Geometry: final body of the model. Coordinates: model frame, mm. A direction names the side the tool comes from. Give positions to 0.01 mm unless a question says otherwise; leave off trailing zeros. Loops run counter-clockwise (first coordinate to the right, second up) from the corner with the lowest first, then second, coordinate; pieces in that order, holes last. Notation, with made-up numbers: (-18, 61.25) -> (-2, 61.25) arc R36 cw to (-2, 99.25) -> close; hole circle Ø2 at (66.25, 63.5). An arc over 180 degrees is marked (long way). One line per question, with ' | ' between items. Start each with the question number.
Item 1: Section B-B on x = 9.5. Return loops of the section in (y, z), then the cut area to 3 significant figures.
Item 2: Section D-D on z = -180. Return loops of the section in (x, y), then the cut area to 3 significant figures.
Item 3: Pin query (flat end, axial travel): P1, Ø1.8, axis at x = -26.5, z = -94, coming from the +Y side; P2, Ø10, axis at y = 37, z = -14.5, coming from the +X side; P3, Ø2, axis at y = 85, z = -59.5, coming from the +X side. Return the tip coordinate at first contact, or that it passes through.
Item 4: Set-up query: faces 1 (the flat face through (7, 56, -137.408)), 2 (the flat face through (-23, 0, 0)). Return all of +Z, -Z, +X, -X, +Y, -Y with unobstructed straight access to the full face (end or side cutting, diameter ignored); none if empty.
Item 5: Section A-A on y = 31. Return loops of the section in (x, z), then the cut area to 3 significant figures.
Item 6: Material intervals for line 1 along X through (y, z) = (23.5, -145.5); line 2 along Y through (x, z) = (-6, -118.5); line 3 along Z through (x, y) = (74, 25.5), sorted ascending. Write a range as [from, to].
Item 7: Section C-C on y = 98. Give the number of separate pieces and of enclosed holes in the cut face, then the cut area to 3 significant figures.
from build123d import *

# Parameters (mm, degrees)
ALUMINUM_BLOCK_DEPTH = 113.03
A_ARM_SKETCHES_R     = 3
A_ARM_HOLES_DEPTH    = 20


with BuildPart() as part:
    # Sketch1 → ALUMINUM BLOCK (new body)
    with BuildSketch(Plane(origin=(0, 0, 0), x_dir=(1, 0, 0), z_dir=(0, 1, 0))):
        Polygon((-187.5, -135.642424533), (244.3, -135.642424533), (244.3, -46.742424533), (98.25, 137.407575467), (-85.9, 137.407575467), (-85.9, 207.257575467), (-187.5, 207.257575467), align=None)
    extrude(amount=ALUMINUM_BLOCK_DEPTH)

    # A-ARM SKETCHES → A-ARM HOLES (cut)
    with BuildSketch(Plane(origin=(0, 113.03, 0), x_dir=(1, 0, 0), z_dir=(0, 1, 0))):
        with Locations(Location((-163.609115423, 145.695818662, 0), (0, 0, 270))):
            Circle(A_ARM_SKETCHES_R)
        with Locations(Location((-3.898882545, 120.015251172, 0), (0, 0, 270))):
            Circle(A_ARM_SKETCHES_R)
        with Locations(Location((175.311223127, -113.149569553, 0), (0, 0, 270))):
            Circle(A_ARM_SKETCHES_R)
        with Locations(Location((-160.15888427, -90.036396379, 0), (0, 0, 270))):
            Circle(A_ARM_SKETCHES_R)
        with Locations(Location((-159.322465718, -117.822298669, 0), (0, 0, 270))):
            Circle(A_ARM_SKETCHES_R)
        with Locations(Location((-120.450372331, -115.251672549, 0), (0, 0, 270))):
            Circle(A_ARM_SKETCHES_R)
        with Locations(Location((-58.544962433, 112.036813196, 0), (0, 0, 270))):
            Circle(A_ARM_SKETCHES_R)
        with Locations(Location((65.478811369, -102.10088587, 0), (0, 0, 270))):
            Circle(A_ARM_SKETCHES_R)
        with Locations(Location((163.603739253, 0.788099457, 0), (0, 0, 270))):
            Circle(A_ARM_SKETCHES_R)
        with Locations(Location((161.606684995, -118.729685562, 0), (0, 0, 270))):
            Circle(A_ARM_SKETCHES_R)
        with Locations(Location((-140.251816154, -97.517207608, 0), (0, 0, 270))):
            Circle(A_ARM_SKETCHES_R)
        with Locations(Location((17.394243717, 117.626925231, 0), (0, 0, 270))):
            Circle(A_ARM_SKETCHES_R)
        with Locations(Location((-26.908089244, 94.447121648, 0), (0, 0, 270))):
            Circle(A_ARM_SKETCHES_R)
    extrude(amount=-A_ARM_HOLES_DEPTH, mode=Mode.SUBTRACT)


solid = part.part
Result sheet:
1) outline: (0, -137.41) -> (113.03, -137.41) -> (113.03, 135.64) -> (0, 135.64) -> close | area: 30,900 mm²
2) outline: (-187.5, 0) -> (-85.9, 0) -> (-85.9, 113.03) -> (-187.5, 113.03) -> close | area: 11,500 mm²
3) P1: stops at y = 93.03 | P2: stops at x = 199.69 | P3: stops at x = 160.83
4) face 1: -Z, +X, +Y, -Y | face 2: +Z, -Z, +X, -X, -Y
5) outline: (-187.5, -207.26) -> (-85.9, -207.26) -> (-85.9, -137.41) -> (98.25, -137.41) -> (244.3, 46.74) -> (244.3, 135.64) -> (-187.5, 135.64) -> close | area: 112,000 mm²
6) line 1: x = [-187.5, -85.9] | line 2: y = [0, 93.03] | line 3: z = [-137.41, 135.64]
7) separate pieces: 1 | enclosed holes: 13 | area: 111,000 mm²
